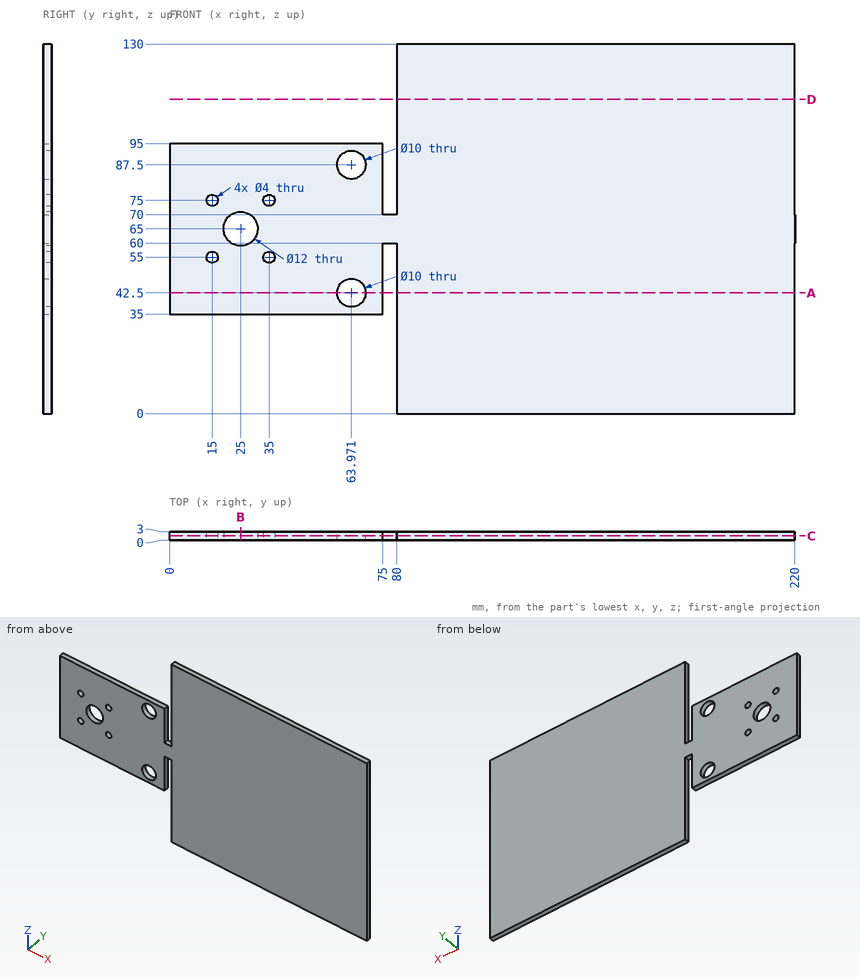
Input: dimensioned drawing with shaded views. Units: mm. Origin: part minimum x, y, z. Give positions to 0.01 mm unless a question says otherwise; leave off trailing zeros. Loops run counter-clockwise (first coordinate to the right, second up) from the corner with the lowest first, then second, coordinate; pieces in that order, holes last. Notation, with made-up numbers: M -31,-35 L 10,-35 A16 cw 10,-26 Z; hole C -15,-29.75 d4. An arc over 180 degrees is marked long. Put each result on its own line as item: value. Start each with the question number.
1) Cut plane A-A (z = 42.5). Output: boundary loops of the cut face in (x, y), then the cut area to 3 significant figures.
2) Ray query, line 1 along X through (y, z) = (0.9, 87.5); line 2 along Z through (x, y) = (35, 1.65); line 3 along X through (y, z) = (1.65, 55). Return the intervals inside material, ascending.
3) Cut plane D-D (z = 110.5). Output: boundary loops of the cut face in (x, y), then the cut area to 3 significant figures.
4) Cut plane B-B (x = 25). Output: boundary loops of the cut face in (y, z).
5) Contact query for flat-ended pins moving along their axis: pin 1 (11 mm diameter, centred on x = 25, z = 65, fed in from +Y) (1 decimal); pin 2 (0.9 mm diameter, centred on x = 19, y = 1.5, fed in from -Z); pin 3 (1.5 mm diameter, centred on x = 55.5, y = 1, fed in from +Z); pin 4 (0.9 mm diameter, centred on y = 1, z = 25.5, fed in from -X). Output: stop coordinate, or through.
6) Cut plane C-C (y = 1.5). Output: boundary loops of the cut face in (x, z), then the cut area to 3 significant figures.
Verdict:
1. outline: M 0,0 L 58.97,0 L 58.97,3 L 0,3 Z; M 68.97,0 L 75,0 L 75,3 L 68.97,3 Z; M 80,0 L 220,0 L 220,3 L 80,3 Z
1. area: 615 mm2
2. line 1: 0 to 58.97, 68.97 to 75, 80 to 220
2. line 2: 35 to 53, 57 to 73, 77 to 95
2. line 3: 0 to 13, 17 to 33, 37 to 75, 80 to 220
3. outline: M 80,0 L 220,0 L 220,3 L 80,3 Z
3. area: 420 mm2
4. outline: M 0,35 L 3,35 L 3,59 L 0,59 Z; M 0,71 L 3,71 L 3,95 L 0,95 Z
5. pin 1: through
5. pin 2: z = 35
5. pin 3: z = 95
5. pin 4: x = 80
6. outline: M 0,35 L 75,35 L 75,60 L 80,60 L 80,0 L 220,0 L 220,130 L 80,130 L 80,70 L 75,70 L 75,95 L 0,95 Z; hole C 15,55 d4; hole C 15,75 d4; hole C 25,65 d12; hole C 35,55 d4; hole C 35,75 d4; hole C 63.97,42.5 d10; hole C 63.97,87.5 d10
6. area: 22,400 mm2
